Geometry: see drawing. Coordinates: mm, zero at the bounding-box minimum. A direction names the side the tool comes from. Coordinates: 2 decimals unless noted, no trailing zeros. Order: outer loops, then holes, each group sorted by start corner. A loop starts at its lowest first (then second) coordinate and runs counter-clockwise, first axis right, second up.
Item 1: Ray query, line 1 (X direction, y = 7, z = 2.5); line 2 (Y direction, x = 44, z = 2.1); line 3 (Z direction, x = 32.5, y = 45.5). Return the intervals inside material, ascending.
Item 2: Section C-C on x = 2.5. Return the cut outline in (y, z), then the cut area to 3 significant figures.
Item 3: Contact query for flat-ended pins moving along their axis: P1, Ø0.5, axis at x = 31, z = 1.5, coming from the +Y side; P2, Ø1.5, axis at y = 42.5, z = 3, coming from the -X side; P3, Ø3, axis at x = 32, y = 31, coming from the +Z side. Output: stop coordinate, or through.
Item 4: Mould query, pull axis Y, two halves, no side actions, for the marked faces 5, 6 and 7. Classes: released by +Y, released by -Y, zero draft, split by the parting line, or undercut.
Item 5: Section D-D on y = 45. Return the cut outline in (x, z).
Item 6: Section A-A on x = 39. Return the cut outline in (y, z).
Item 7: Section B-B on y = 10.5. Return the cut outline in (x, z).
Item 8: Reachability of the marked faces 1, 2, 3 and 4 from +Z, -Z, +X, -X, +Y, -Y: full face, straight path, thin tool, end or side. Return the list, or none.
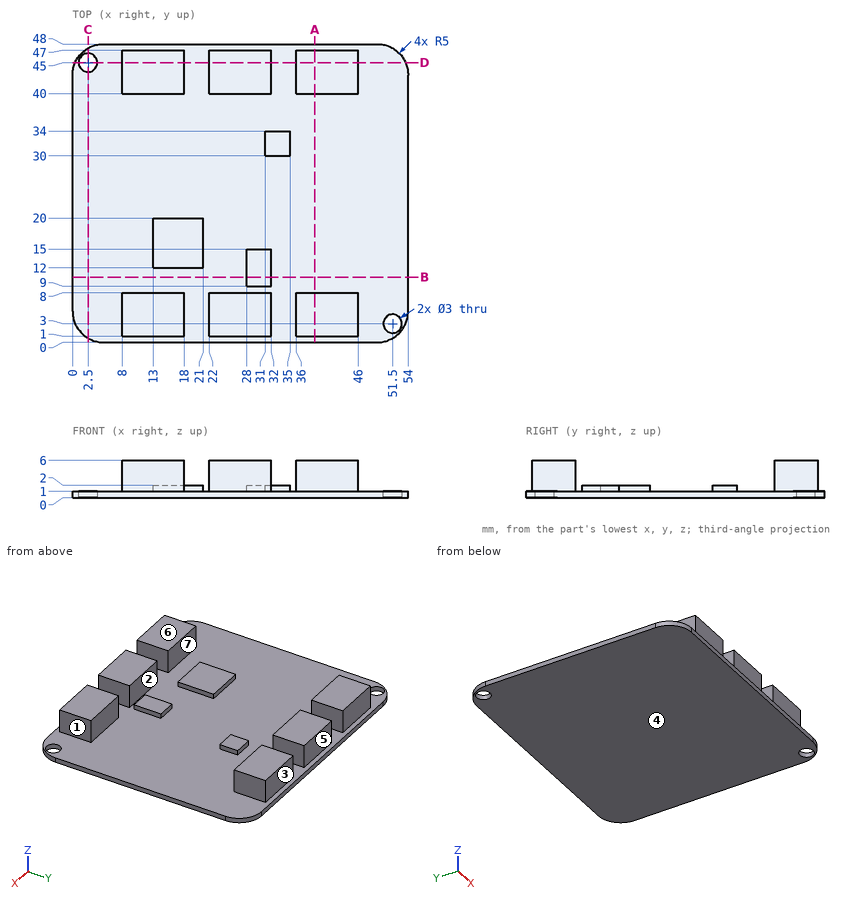
Answer list:
1. line 1: x = 8 to 18, 22 to 32, 36 to 46
1. line 2: y = 1 to 8, 40 to 47
1. line 3: z = 0 to 1
2. outline: (0.67, 0) - (43.5, 0) - (43.5, 1) - (0.67, 1) - close; (46.5, 0) - (47.33, 0) - (47.33, 1) - (46.5, 1) - close
2. area: 43.7 mm2
3. P1: stops at y = 47
3. P2: stops at x = 8
3. P3: stops at z = 2
4. face 5: released by +Y
4. face 6: zero draft
4. face 7: undercut
5. outline: (0.42, 0) - (1, 0) - (1, 1) - (0.42, 1) - close; (4, 0) - (53.58, 0) - (53.58, 1) - (46, 1) - (46, 6) - (36, 6) - (36, 1) - (32, 1) - (32, 6) - (22, 6) - (22, 1) - (18, 1) - (18, 6) - (8, 6) - (8, 1) - (4, 1) - close
6. outline: (0, 0) - (48, 0) - (48, 1) - (47, 1) - (47, 6) - (40, 6) - (40, 1) - (8, 1) - (8, 6) - (1, 6) - (1, 1) - (0, 1) - close
7. outline: (0, 0) - (54, 0) - (54, 1) - (32, 1) - (32, 2) - (28, 2) - (28, 1) - (0, 1) - close
8. face 1: +Z, +X, +Y, -Y
8. face 2: +Z, +X, -X
8. face 3: +Z, +X, -X, +Y
8. face 4: -Z, +X, -X, +Y, -Y
